Build history of the part. All positions in model axes, mm. A direction names the side the tool comes from. Coordinates: 2 decimals unless noted, no trailing zeros. Loops run counter-clockwise (first coordinate to the right, second up) from the corner with the lowest first, then second, coordinate; pieces in that order, holes last. Notation, with made-up numbers: M 36.25,80.5 L 67.25,80.5 A24 ccw 67.25,102.5 Z; hole C 36.5,-5.5 d8. An arc over 180 degrees is marked long. Write each question's results on one line, items separated by ' | '. Start each with the question number.
from build123d import *

# Parameters (mm, degrees)
BEARING_HOUSING_PROFILE_R                  = 17
BEARING_HOUSING_PROFILE_R_2                = 11.1
BEARING_HOUSING_DEPTH                      = 7
MOUNTING_WEB_PROFILE_W                     = 30
MOUNTING_WEB_PROFILE_H                     = 28
MOUNTING_WEB_DEPTH                         = 4
BEARING_SEAT_START                         = -50
BEARING_SEAT_PROFILE_R                     = 11.1
BEARING_SEAT_DEPTH                         = 86.185224172
INNER_OUTER_RACE_RETAINING_LIP_START       = -1
INNER_OUTER_RACE_RETAINING_LIP_PROFILE_R   = 17
INNER_OUTER_RACE_RETAINING_LIP_PROFILE_R_2 = 9
INNER_OUTER_RACE_RETAINING_LIP_DEPTH       = 1
STANDOFF_FASTENERS_START                   = -50
STANDOFF_FASTENERS_PROFILE_R               = 1.6
STANDOFF_FASTENERS_DEPTH                   = 86.185224172
BEARING_KEEPER_FASTENERS_START             = -50
BEARING_KEEPER_FASTENERS_PROFILE_R         = 1.1
BEARING_KEEPER_FASTENERS_DEPTH             = 86.185224172
FILLET1_R                                  = 3


with BuildPart() as part:
    # Bearing_housing_profile → Bearing_housing (new body)
    with BuildSketch(Plane.XY):
        Circle(BEARING_HOUSING_PROFILE_R)
        Circle(BEARING_HOUSING_PROFILE_R_2, mode=Mode.SUBTRACT)
    extrude(amount=BEARING_HOUSING_DEPTH)

    # Mounting_web_profile → Mounting_web (add)
    with BuildSketch(Plane.XY):
        with Locations((-15, 0)):
            Rectangle(MOUNTING_WEB_PROFILE_W, MOUNTING_WEB_PROFILE_H)
    extrude(amount=MOUNTING_WEB_DEPTH)

    # Bearing_seat_profile → Bearing_seat (cut, through all)
    with BuildSketch(Plane.XY.offset(BEARING_SEAT_START)):
        Circle(BEARING_SEAT_PROFILE_R)
    extrude(amount=BEARING_SEAT_DEPTH, mode=Mode.SUBTRACT)

    # Inner_outer_race_retaining_lip_profile → Inner_outer_race_retaining_lip (add)
    with BuildSketch(Plane.XY.offset(INNER_OUTER_RACE_RETAINING_LIP_START)):
        Circle(INNER_OUTER_RACE_RETAINING_LIP_PROFILE_R)
        Circle(INNER_OUTER_RACE_RETAINING_LIP_PROFILE_R_2, mode=Mode.SUBTRACT)
    extrude(amount=INNER_OUTER_RACE_RETAINING_LIP_DEPTH)

    # Standoff_fasteners_profile → Standoff_fasteners (cut, through all)
    with BuildSketch(Plane.XY.offset(STANDOFF_FASTENERS_START)):
        with Locations(Location((-25, -9, 0), (0, 0, 180))):
            Circle(STANDOFF_FASTENERS_PROFILE_R)
        with Locations(Location((-25, 9, 0), (0, 0, 180))):
            Circle(STANDOFF_FASTENERS_PROFILE_R)
    extrude(amount=STANDOFF_FASTENERS_DEPTH, mode=Mode.SUBTRACT)

    # Bearing_keeper_fasteners_profile → Bearing_keeper_fasteners (cut, through all)
    with BuildSketch(Plane.XY.offset(BEARING_KEEPER_FASTENERS_START)):
        with Locations(Location((14, 0, 0), (0, 0, 180))):
            Circle(BEARING_KEEPER_FASTENERS_PROFILE_R)
        with Locations(Location((0, -14, 0), (0, 0, 180))):
            Circle(BEARING_KEEPER_FASTENERS_PROFILE_R)
        with Locations(Location((0, 14, 0), (0, 0, 180))):
            Circle(BEARING_KEEPER_FASTENERS_PROFILE_R)
    extrude(amount=BEARING_KEEPER_FASTENERS_DEPTH, mode=Mode.SUBTRACT)

    # Fillet1
    fillet1_edges = [part.edges().sort_by_distance(p)[0] for p in [
        (-30, -14, 2),
        (-30, 14, 2),
    ]]
    fillet(fillet1_edges, radius=FILLET1_R)


solid = part.part
1. Band-saw the part on B-B, the plane x = -25. List the corners of the cut face in (y, z), plus the area to 3 significant figures.
2. Wall check: line 1 along Y through (x, z) = (0, 3.75); line 2 along Y through (x, z) = (-25, 1.35); line 3 along Y through (x, z) = (0, -0.5). Give the ranges that are in metal, low to high.
3. Which spindle directions (+Z, -Z, +X, -X, +Y, -Y) get a long thin tool onto all of the face, cutting with end or side? Do faces 1 (the flat face through (-2, 9, 0)), 2 (the cylindrical face through (-1.172, 8.923, -0.507)), 3 (the flat face through (-18, -14, 2)), 4 (the flat face through (-30, 0, 2)), 5 (the flat face through (-18, 14, 2)). Say none if no direction does.
4. Pin check, flat tips, straight feed: pin 1 (4 mm diameter, centred on x = 9.5, z = 3, fed in from -Y); pin 2 (4 mm diameter, centred on x = -21.5, y = 7, fed in from -Z); pin 3 (5 mm diameter, centred on x = -25, y = -9, fed in from +Z); pin 4 (1.8 mm diameter, centred on x = 0, y = -14, fed in from -Z). Stop position of each tip, or through.
5. Band-saw the part on D-D, the plane x = 0. List the corners of the cut face in (y, z), plus the area to 3 significant figures.
6. Band-saw the part on C-C, the plane z = 1.5. List the corners of the cut face in (x, y).
7. Band-saw the part on A-A, the plane y = 0. List the corners of the cut face in (x, z), plus the area to 3 significant figures.
8. Mould opens along Y. For faces 6 (the cylindrical face through (5.97, 9.36, 3.45)), 7 (the cylindrical face through (-29.1, 13.14, 2.03)), 8 (the flat face through (-22, 0, 4)) say: +Y half, -Y half, draft (parallel to the pull), parting line (faces both ways), or undercut.
Checked values:
1) outline: M -14,0 L -10.6,0 L -10.6,4 L -14,4 Z; M -7.4,0 L 7.4,0 L 7.4,4 L -7.4,4 Z; M 10.6,0 L 14,0 L 14,4 L 10.6,4 Z | area: 86.4 mm²
2) line 1: -17 to -15.1, -12.9 to -11.1, 11.1 to 12.9, 15.1 to 17 | line 2: -14 to -10.6, -7.4 to 7.4, 10.6 to 14 | line 3: -17 to -15.1, -12.9 to -9, 9 to 12.9, 15.1 to 17
3) face 1: +Z | face 2: +Z, -Z | face 3: +Z, -Z, -X, -Y | face 4: +Z, -Z, -X, +Y, -Y | face 5: +Z, -Z, -X, +Y
4) pin 1: y = -15.26 | pin 2: z = 0 | pin 3: z = 4 | pin 4: through
5) outline: M -17,-1 L -15.1,-1 L -15.1,7 L -17,7 Z; M -12.9,-1 L -9,-1 L -9,0 L -11.1,0 L -11.1,7 L -12.9,7 Z; M 9,-1 L 12.9,-1 L 12.9,7 L 11.1,7 L 11.1,0 L 9,0 Z; M 15.1,-1 L 17,-1 L 17,7 L 15.1,7 Z | area: 63.4 mm²
6) outline: M -30,-11 A3 ccw -27,-14 L -9.64,-14 A17 ccw long -9.64,14 L -27,14 A3 ccw -30,11 Z; hole C -25,-9 d3.2; hole C -25,9 d3.2; hole C 0,0 d22.2; hole C 0,-14 d2.2; hole C 0,14 d2.2; hole C 14,0 d2.2
7) outline: M -30,0 L -17,0 L -17,-1 L -9,-1 L -9,0 L -11.1,0 L -11.1,7 L -17,7 L -17,4 L -30,4 Z; M 9,-1 L 12.9,-1 L 12.9,7 L 11.1,7 L 11.1,0 L 9,0 Z; M 15.1,-1 L 17,-1 L 17,7 L 15.1,7 Z | area: 133 mm²
8) face 6: undercut | face 7: +Y half | face 8: draft
